Autodesk Inventor part; units mm, degrees
ref_plane "YZ Plane" through (0, 0, 0) normal (1, 0, 0) x (0, 1, 0)
ref_plane "XZ Plane" through (0, 0, 0) normal (0, 1, 0) x (-1, 0, 0)
ref_plane "XY Plane" through (0, 0, 0) normal (0, 0, 1) x (1, 0, 0)
sketch "Sketch1" plane through (0, 0, 0) normal (0, 1, 0) x (-1, 0, 0)
  line L0 (0, 0) -> (26.25, 0) construction
  line L1 (26.25, 0) -> (26.25, -22) construction
  line L2 (26.25, -22) -> (0, -22) construction
  line L3 (0, -22) -> (0, 0) construction
  circle A0 centre (2, -20) radius 1.95
  circle A1 centre (24.25, -2) radius 2
  dimension "d0" = 26.25
  dimension "d1" = 22
  dimension "d3" = 3.9
  dimension "d6" = 4
  dimension "d18" = 2
  dimension "d19" = 2
  dimension "d20" = 2
  dimension "d21" = 2
extrude "Extrusion1" add sketch "Sketch1" along normal blind 2.8
sketch "Sketch6" plane through (-24.25, 0, -2) normal (0, -1, 0) x (1, 0, 0)
  circle A0 centre (0, 0) radius 2 construction
  circle A1 centre (22.25, -18) radius 1.95 construction
  line L0 (-7.7702, -20) -> (30.063, -20) construction
  line L1 (1.9389, 3.3329) -> (25.6312, -15.8338)
  line L2 (25.6312, -15.8338) -> (25.6312, -20)
  circle A2 centre (22.25, -18) radius 1.95
  line L3 (4, -20) -> (4, -16)
  line L4 (4, -16) -> (12.25, -16)
  line L5 (12.25, -16) -> (12.25, -20)
  line L6 (25.6312, -20) -> (12.25, -20)
  line L7 (4, -20) -> (-3.1908, -20)
  line L8 (2.5513, -5.9922) -> (9.3088, -11.459)
  line L9 (9.3088, -11.459) -> (2.5513, -11.459)
  line L10 (2.5513, -11.459) -> (2.5513, -5.9922)
  line L11 (-3.1908, -20) -> (-3.1908, 3.3329)
  line L12 (1.9389, 3.3329) -> (-3.1908, 3.3329)
  point P0 (24.25, 2)
  dimension "d28" = 2
  dimension "d31" = 10
  dimension "d32" = 4
  dimension "d40" = 4
extrude "Extrusion6" add sketch "Sketch6" along normal blind 2.5 contours L1 L2 L6 L5 L4 L3 L7 L11 L12 | A2
fillet "Fillet1" radius 2 1 edges at (-22.25, 0, -2)
hole "Hole1" at (-24.25, 2.8, -2) direction (0, -1, 0) diameter 2 depth 8 tip angle 118
hole "Hole2" at (-2, 2.8, -20) direction (0, -1, 0) diameter 2 depth 8 tip angle 118
fillet "Fillet2" radius 2 1 edges at (-0.05, 0, -20)
sketch "Sketch10" plane through (1.3812, -2.5, -22) normal (0, 0, -1) x (-1, 0, 0)
  line L0 (25.6312, -4.2658) -> (25.6312, 25.595) construction
  line L1 (3.3812, -4.2658) -> (3.3812, 25.595) construction
  line L2 (0, 0) -> (23.6922, 0)
  line L3 (3.3812, 0) -> (25.6312, 0)
  line L4 (25.6312, 0) -> (25.6312, 21.3292)
  line L5 (25.6312, 21.3292) -> (3.3812, 21.3292)
  line L6 (3.3812, 21.3292) -> (3.3812, 0)
  point P0 (1.3812, 2.5)
extrude "Extrusion8" add sketch "Sketch10" along normal blind 3
fillet "Fillet3" radius 2 1 edges at (-2, -0.4722, -22)
fillet "Fillet4" radius 2 1 edges at (-24.25, -1.25, -22)
fillet "Fillet5" radius 2 1 edges at (-22.25, 0, -22)
sketch "Sketch12" plane through (1.3812, -2.5, -22) normal (0, 0, 1) x (1, 0, 0)
  line L0 (-23.6312, 5.3) -> (-27.6312, 5.3) construction
  line L1 (-1.4312, 5.3) -> (-5.3312, 5.3) construction
  circle A0 centre (-20.5062, 18.3) radius 2
  circle A1 centre (-20.5062, 10.3) radius 2
  line L2 (-25.6312, 4.5) -> (-25.6312, 21.3292)
  line L3 (-3.3812, 21.3292) -> (-3.3812, 0) construction
  line L4 (-3.3812, 12.9146) -> (-25.6312, 12.9146) construction
  line L5 (-14.5062, 12.9146) -> (-14.5062, 6.5641) construction
  circle A2 centre (-8.5062, 18.3) radius 2
  circle A3 centre (-8.5062, 10.3) radius 2
  point P0 (-1.3812, 2.5)
  dimension "d67" = 4
  dimension "d70" = 5.125
  dimension "d72" = 5
  dimension "d73" = 5.125
  dimension "d112" = 12
  dimension "d113" = 8
extrude "Extrusion9" cut sketch "Sketch12" against normal blind 0.3
hole "Hole3" at (-19.125, 7.8, -22.3) direction (0, 0, -1) diameter 2 depth 8 tip angle 118
hole "Hole4" at (-19.125, 15.8, -22.3) direction (0, 0, -1) diameter 2 depth 8 tip angle 118
hole "Hole5" at (-7.125, 15.8, -22.3) direction (0, 0, -1) diameter 2 depth 8 tip angle 118
hole "Hole6" at (-7.125, 7.8, -22.3) direction (0, 0, -1) diameter 2 depth 8 tip angle 118
ref_plane "Work Plane3" through (-13.125, 7.8, -26.3) normal (-1, 0, 0) x (0, 0, 1)
ref_plane "Work Plane1" through (-7.125, 15.8, -26.3) normal (1, 0, 0) x (0, 0, 1)
ref_plane "Work Plane2" through (-19.125, 7.8, -26.3) normal (-1, 0, 0) x (0, 0, 1)
sketch "Sketch14" plane through (-24.25, 18.8292, -22) normal (0, 1, 0) x (1, 0, 0)
  line L0 (22.25, 0) -> (0, 0)
  line L1 (0, 0) -> (0, 3)
  line L2 (22.25, 3) -> (0, 3)
  line L3 (22.25, 3) -> (22.25, 0)
  arc A0 (0, 3) -> (22.25, 3) centre (11.125, -42.8915) ccw
  point P0 (24.25, -22)
extrude "Extrusion11" cut sketch "Sketch14" against normal through all contours L3 A0 L1 L0
sketch "Sketch15" plane through (-24.25, -2.5, -2) normal (0, -1, 0) x (1, 0, 0)
  line L0 (-3.375, -6) -> (25.625, -6)
  line L1 (25.625, -6) -> (25.625, -23)
  line L2 (25.625, -23) -> (-3.375, -23)
  line L3 (-3.375, -23) -> (-3.375, -6)
  line L4 (22.25, -20) -> (0, -20) construction
  line L5 (11.125, -28) -> (11.125, 7) construction
  line L6 (0, -20) -> (22.25, -20) construction
  line L7 (22.25, -23) -> (0, -23)
  point P0 (24.25, 2)
  point P1 (11.125, -23)
  point P2 (11.125, -20)
  point P3 (11.125, -20)
  point P4 (11.125, -23)
  point P5 (11.125, -23)
  dimension "d128" = 29
  dimension "d129" = 17
extrude "Extrusion12" add sketch "Sketch15" along normal blind 1.5 and the other way blind 1
sketch "Sketch19" plane through (-24.25, -1.5, -2) normal (0, 1, 0) x (1, 0, 0)
  circle A0 centre (22.125, 9.8) radius 2.25
  circle A1 centre (0.125, 9.8) radius 2.25
  line L0 (0.125, 9.8) -> (22.125, 9.8) construction
  line L1 (11.125, -7) -> (11.125, 28) construction
  line L2 (0, 20) -> (22.25, 20) construction
  line L3 (0, 20) -> (22.25, 20) construction
  line L4 (19.125, 20) -> (15.125, 20) construction
  line L5 (7.125, 20) -> (3.125, 20) construction
  line L6 (7.125, 20) -> (3.125, 20) construction
  line L7 (19.125, 20) -> (15.125, 20) construction
  point P0 (24.25, -2)
  point P1 (11.125, 9.8)
  dimension "d154" = 4.5
  dimension "d155" = 4.5
  dimension "d156" = 22
  dimension "d157" = 10.2
extrude "Extrusion16" add sketch "Sketch19" along normal blind 1.35
sketch "Sketch16" plane through (-24.25, -4, -2) normal (0, -1, 0) x (1, 0, 0)
  line L0 (15.125, -20) -> (19.125, -20) construction
  line L1 (3.125, -20) -> (7.125, -20) construction
  line L2 (3.125, -20) -> (7.125, -20) construction
  line L3 (15.125, -20) -> (19.125, -20) construction
  line L4 (0, -20) -> (22.25, -20) construction
  line L5 (0, -20) -> (22.25, -20) construction
  line L6 (0, -23) -> (0, -20) construction
  line L7 (22.25, -20) -> (22.25, -23) construction
  line L8 (11.125, -28) -> (11.125, 7) construction
  circle A0 centre (0.125, -9.8) radius 1
  circle A1 centre (22.125, -9.8) radius 1
  line L9 (0.125, -9.8) -> (22.125, -9.8) construction
  point P0 (24.25, 2)
  point P1 (11.125, -9.8)
  dimension "d132" = 2
  dimension "d133" = 2
  dimension "d134" = 22
  dimension "d135" = 10.2
extrude "Extrusion13" cut sketch "Sketch16" against normal through all
sketch "Sketch17" plane through (-24.25, -4, -2) normal (0, -1, 0) x (1, 0, 0)
  line L0 (15.125, -20) -> (19.125, -20) construction
  line L1 (3.125, -20) -> (7.125, -20) construction
  line L2 (3.125, -20) -> (7.125, -20) construction
  line L3 (15.125, -20) -> (19.125, -20) construction
  line L4 (0, -20) -> (22.25, -20) construction
  line L5 (0, -20) -> (22.25, -20) construction
  line L6 (22.25, -20) -> (22.25, -23) construction
  line L7 (22.25, -20) -> (22.25, -23) construction
  line L8 (0, -20) -> (0, -23) construction
  line L9 (0, -23) -> (0, -20) construction
  line L10 (3.875, -2.15) -> (7.875, -2.15)
  line L11 (7.875, -2.15) -> (7.875, -11.65)
  line L12 (7.875, -11.65) -> (3.875, -11.65)
  line L13 (3.875, -11.65) -> (3.875, -2.15)
  circle A0 centre (22.125, -9.8) radius 1
  line L14 (17.425, -10.6) -> (20.425, -10.6)
  line L15 (20.425, -10.6) -> (20.425, -16.6)
  line L16 (20.425, -16.6) -> (17.425, -16.6)
  line L17 (17.425, -16.6) -> (17.425, -10.6)
  circle A1 centre (0.125, -9.8) radius 1
  point P0 (24.25, 2)
  dimension "d138" = 9.5
  dimension "d139" = 4
  dimension "d142" = 6
  dimension "d143" = 3
  dimension "d161" = 3.75
  dimension "d162" = 1.7
  dimension "d163" = 3.4
  dimension "d164" = 8.35
extrude "Extrusion14" cut sketch "Sketch17" against normal through all contours L10 L11 L12 L13 | L14 L15 L16 L17
fillet "Fillet9" radius 2 4 edges at (1.375, -2.75, -25) (1.375, -2.75, -8) (-27.625, -2.75, -8) (-27.625, -2.75, -25)
fillet "Fillet10" radius 2 2 edges at (-2, -1.5, -23.5) (-24.25, -1.5, -23.5)
sketch "Sketch20" plane through (-24.25, -4, -2) normal (0, -1, 0) x (1, 0, 0)
  line L0 (24.25, -20) -> (-2, -20) construction
  line L1 (22.25, -20) -> (24.25, -20) construction
  line L2 (0, -20) -> (22.25, -20) construction
  line L3 (-2, -20) -> (0, -20) construction
  line L4 (15.125, -20) -> (19.125, -20) construction
  line L5 (3.125, -20) -> (7.125, -20) construction
  line L6 (3.125, -20) -> (7.125, -20) construction
  line L7 (15.125, -20) -> (19.125, -20) construction
  line L8 (0, -20) -> (0, -23) construction
  line L9 (0, -20) -> (0, -23) construction
  line L10 (22.25, -23) -> (22.25, -20) construction
  line L11 (22.25, -20) -> (22.25, -23) construction
  line L12 (4.8017, -16.5933) -> (11.8961, -13.2182)
  line L13 (11.8961, -13.2182) -> (12.8095, -15.138)
  line L14 (12.8095, -15.138) -> (5.7151, -18.5131)
  line L15 (5.7151, -18.5131) -> (4.8017, -16.5933)
  point P0 (24.25, 2)
extrude "Extrusion17" cut sketch "Sketch20" against normal through all
properties part number "camera_support_.Fatshark_600TVLipt" material "ABS Plastic"
Here's how the part is built. I have some questions about the finished solid (model axes, mm). A direction names the side the tool comes from. Round coordinates to 2 decimals unless told otherwise and drop trailing zeros. Loops run counter-clockwise (first coordinate to the right, second up) from the corner with the lowest first, then second, coordinate; pieces in that order, holes last.
1. If I drill on probe 1 along X at (y, z) = (15.8, -23.5) (3 decimals); probe 2 along X at (y, z) = (-2.5, -14.5) (3 decimals); probe 3 along Y at (x, z) = (-6.25, -11.5), over which ranges is the centre line in solid material (lowest first)?
Answers:
probe 1: x = -24.25 to -20.125, -18.125 to -8.125, -6.125 to -2
probe 2: x = -27.625 to -6.825, -3.825 to 1.375
probe 3: y = -4 to -1.5
2. For faces 4 (the face through (-5, -3, -18.6)), 5 (the face through (-19, 17, -22.3)), 6 (the face through (-23.09, -0.83, -13.8)), 7 (the face through (-20.375, -3, -11)), 8 (the face through (-23, -0.15, -11)), which set-ups out of +Z, -Z, +X, -X, +Y, -Y let a thin tool reach every point of the face, with its end or its side?
Answers:
face 4: +Y, -Y
face 5: +Z
face 6: +Y
face 7: +Z, +Y, -Y
face 8: +Z, +X, -X, +Y
3. Suppose I cut it at C-C, the plane z = -23.5. Give the number of separate pieces and of enclosed holes in the cut face, and give its area (3 significant figures).
Answers:
separate pieces: 1
enclosed holes: 4
area: 514 mm2
4. Will these pins go through, and if not, where does the flat tip stop? pin 1 (3.5 mm diameter, centred on x = -23, z = -13, fed in from +Y); pin 2 (1.8 mm diameter, centred on x = -7.125, y = 15.8, fed in from +Z); pin 3 (2.5 mm diameter, centred on x = -19.125, y = 15.8, fed in from +Z); pin 4 (5 mm diameter, centred on x = -12.5, y = 15.5, fed in from +Z).
Answers:
pin 1: stops at y = -0.15
pin 2: passes through
pin 3: stops at z = -22.3
pin 4: stops at z = -22
5. Suppose I cut it at B-B, the plane y = 15.8. Please give me the cut outline in (x, z) (3 decimals).
Answers:
outline: (-24.25, -25) - (-20.125, -25) - (-20.125, -22.3) - (-21.125, -22.3) - (-21.125, -22) - (-24.25, -22) - close; (-18.125, -25) - (-8.125, -25) - (-8.125, -22.3) - (-9.125, -22.3) - (-9.125, -22) - (-17.125, -22) - (-17.125, -22.3) - (-18.125, -22.3) - close; (-6.125, -25) - (-2, -25) - (-2, -22) - (-5.125, -22) - (-5.125, -22.3) - (-6.125, -22.3) - close
6. Thinking about a two-plate mould opening in X: for faces 1 (the face through (-20.6, 17.15, -22.15)), 2 (the face through (0.774, -2.732, -8.57)), 3 (the face through (-23, -3, -8)), which applies, released by +X, released by -X, zero draft, split by the parting line, or undercut?
Answers:
face 1: undercut
face 2: released by +X
face 3: zero draft
7. Suppose I cut it at A-A, the plane z = -11.8. Please give me the cut outline in (x, y) (3 decimals).
Answers:
outline: (-27.625, -4) - (-25.125, -4) - (-25.125, -0.15) - (-26.375, -0.15) - (-26.375, -1.5) - (-27.625, -1.5) - close; (-23.125, -4) - (-20.375, -4) - (-20.375, -1.5) - (-21.875, -1.5) - (-21.875, -0.15) - (-23.125, -0.15) - close; (-16.375, -4) - (-3.125, -4) - (-3.125, -0.15) - (-4.375, -0.15) - (-4.375, -1.5) - (-16.375, -1.5) - close; (-1.125, -4) - (1.375, -4) - (1.375, -1.5) - (0.125, -1.5) - (0.125, -0.15) - (-1.125, -0.15) - close
8. Suppose I cut it at D-D, the plane z = -16.5. Please give me the cut outline in (x, y) (3 decimals), and give its area (3 significant figures).
Answers:
outline: (-27.625, -4) - (-15.048, -4) - (-15.048, -1.5) - (-27.625, -1.5) - close; (-11.744, -4) - (-6.825, -4) - (-6.825, -1.5) - (-11.744, -1.5) - close; (-3.825, -4) - (1.375, -4) - (1.375, -1.5) - (-3.825, -1.5) - close
area: 56.7 mm2
